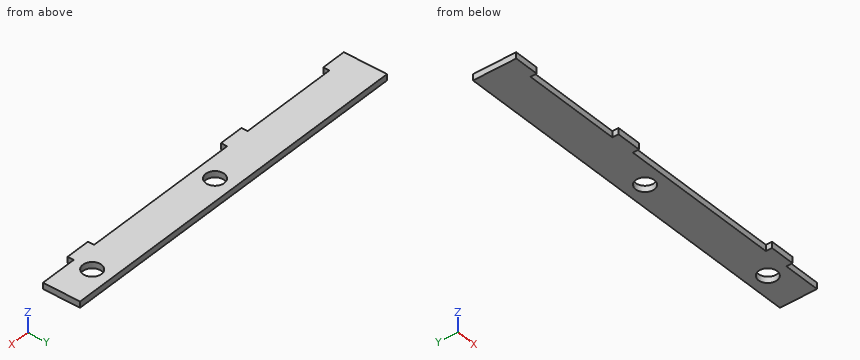
Autodesk Inventor part; units mm, degrees
ref_plane "YZ Plane" through (0, 0, 0) normal (1, 0, 0) x (0, 1, 0)
ref_plane "XZ Plane" through (0, 0, 0) normal (0, 1, 0) x (-1, 0, 0)
ref_plane "XY Plane" through (0, 0, 0) normal (0, 0, 1) x (1, 0, 0)
sketch "Sketch1" plane through (0, 0, 0) normal (0, 0, 1) x (1, 0, 0)
  line L0 (-150, 15) -> (150, 15)
  line L1 (150, 15) -> (150, -15)
  line L2 (150, -15) -> (-150, -15)
  line L3 (-150, -15) -> (-150, 15)
  line L4 (-150, 15) -> (150, -15) construction
  line L5 (150, 15) -> (-150, -15) construction
  point P0 (0, 0)
  dimension "d0" = 300
  dimension "d1" = 30
extrude "Base" add sketch "Sketch1" along normal blind 5
sketch "Sketch2" plane through (0, 0, 5) normal (0, 0, 1) x (1, 0, 0)
  line L0 (-150, -15) -> (150, -15)
  line L1 (-150, -15) -> (-130, -15)
  line L2 (-130, -15) -> (-130, -20)
  line L3 (-130, -20) -> (-150, -20)
  line L4 (-150, -20) -> (-150, -15)
  line L5 (-100, -15) -> (-80, -15)
  line L6 (-80, -15) -> (-80, -20)
  line L7 (-80, -20) -> (-100, -20)
  line L8 (-100, -20) -> (-100, -15)
  line L9 (-50, -15) -> (-30, -15)
  line L10 (-30, -15) -> (-30, -20)
  line L11 (-30, -20) -> (-50, -20)
  line L12 (-50, -20) -> (-50, -15)
  line L13 (0, -15) -> (20, -15)
  line L14 (20, -15) -> (20, -20)
  line L15 (20, -20) -> (0, -20)
  line L16 (0, -20) -> (0, -15)
  line L17 (50, -15) -> (70, -15)
  line L18 (70, -15) -> (70, -20)
  line L19 (70, -20) -> (50, -20)
  line L20 (50, -20) -> (50, -15)
  line L21 (100, -15) -> (120, -15)
  line L22 (120, -15) -> (120, -20)
  line L23 (120, -20) -> (100, -20)
  line L24 (100, -20) -> (100, -15)
  point P0 (0, 0)
  point P1 (20, -15)
  point P2 (0, -15)
  point P3 (-30, -15)
  point P4 (-50, -15)
  point P5 (-130, -15)
  point P6 (70, -15)
  point P7 (50, -15)
  point P8 (-80, -15)
  point P9 (-100, -15)
  point P10 (120, -15)
  point P11 (100, -15)
  dimension "d4" = 20
  dimension "d5" = 5
  dimension "d8" = 50
extrude "Encaixe" add sketch "Sketch2" against normal blind 5 contours L0 L22 L23 L24 | L0 L10 L11 L12 | L0 L2 L3 L4
sketch "Sketch3" plane through (0, 0, 5) normal (0, 0, 1) x (1, 0, 0)
  circle A0 centre (120, 0) radius 7.5
  circle A1 centre (0, 0) radius 7.5
  line L0 (150, -15) -> (150, 15)
  dimension "d16" = 15
  dimension "d17" = 15
  dimension "d20" = 30
extrude "Extrusion3" cut sketch "Sketch3" against normal blind 10
properties part number "Divisória-30cm c rolamento"
Build history of the part. All positions in model axes, mm. Give positions to 0.01 mm unless a question says otherwise; leave off trailing zeros. Order: outer loops, then holes, each group sorted by start corner. A loop starts at its lowest first (then second) coordinate and runs counter-clockwise, first axis right, second up. Notation, with made-up numbers: M -26.75,51.5 L -3.75,51.5 A34 ccw -3.75,90.5 Z; hole C 24.25,10.25 d1. An arc over 180 degrees is marked long. Use one line per item in the form item = value.
1) Saw through at A-A (x = 0). Give the cut face in (y, z).
Calculated:
outline = M -15,0 L -7.5,0 L -7.5,5 L -15,5 Z; M 7.5,0 L 15,0 L 15,5 L 7.5,5 Z
2) Saw through at D-D (x = -53.5). Give the cut face in (y, z), plus the area to 3 significant figures.
Calculated:
outline = M -15,0 L 15,0 L 15,5 L -15,5 Z
area = 150 mm2
3) Saw through at C-C (y = 0). Give the cut face in (x, z), plus the area to 3 significant figures.
Calculated:
outline = M -150,0 L -7.5,0 L -7.5,5 L -150,5 Z; M 7.5,0 L 112.5,0 L 112.5,5 L 7.5,5 Z; M 127.5,0 L 150,0 L 150,5 L 127.5,5 Z
area = 1,350 mm2
4) Drop flat-ended pins along their axis: pin 1 (6 mm diameter, centred on x = -28, y = 6.5, fed in from -Z); pin 2 (1.5 mm diameter, centred on x = 15, z = 2.5, fed in from -Y); pin 3 (1.5 mm diameter, centred on y = -17, z = 2.5, fed in from +X). Give the stop position or say it passes through.
Calculated:
pin_1 = 0
pin_2 = -15
pin_3 = 120
5) Saw through at B-B (z = 1). Give the cut face in (x, y), plus the area to 3 significant figures.
Calculated:
outline = M -150,-20 L -130,-20 L -130,-15 L -50,-15 L -50,-20 L -30,-20 L -30,-15 L 100,-15 L 100,-20 L 120,-20 L 120,-15 L 150,-15 L 150,15 L -150,15 Z; hole C 0,0 d15; hole C 120,0 d15
area = 8,950 mm2
6) Probe probe 1 along X at (y, z) = (0.5, 1.5); probe 2 along X at (y, z) = (-16, 4.85); probe 3 along Y at (x, z) = (0, 1.4). List the from-to ranges inside material, lowest first.
Calculated:
probe_1 = -150 to -7.48, 7.48 to 112.52, 127.48 to 150
probe_2 = -150 to -130, -50 to -30, 100 to 120
probe_3 = -15 to -7.5, 7.5 to 15
